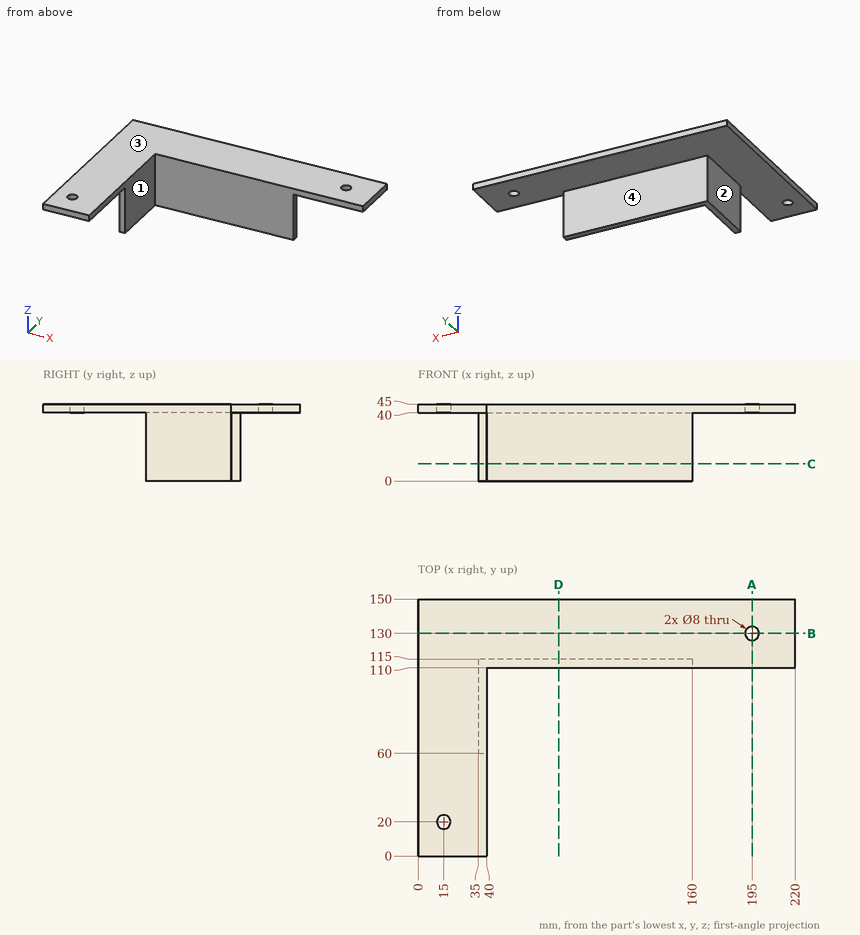
Print and shaded views of the part. All mm, measured from the part's lowest x, y and z. A direction names the side the tool comes from. Give positions to 0.01 mm unless a question says otherwise; leave off trailing zeros. Loops run counter-clockwise (first coordinate to the right, second up) from the corner with the lowest first, then second, coordinate; pieces in that order, holes last. Notation, with made-up numbers: (58.25, 57.25) - (93.25, 57.25) arc R23 cw to (93.25, 82.25) - close; hole circle Ø7 at (-19.75, 58). An arc over 180 degrees is marked (long way). Use a Markdown table: item, result.
(1) Band-saw the part on B-B (y = 130). Give the cut face in (x, z).
Taken from the geometry:
| item | result |
|---|---|
| outline | (0, 40) - (191, 40) - (191, 45) - (0, 45) - close; (199, 40) - (220, 40) - (220, 45) - (199, 45) - close |
(2) Band-saw the part on D-D (x = 82). Give the cut face in (y, z).
Taken from the geometry:
| item | result |
|---|---|
| outline | (110, 0) - (115, 0) - (115, 40) - (150, 40) - (150, 45) - (110, 45) - close |
(3) Band-saw the part on C-C (z = 10). Give the cut face in (x, y).
Taken from the geometry:
| item | result |
|---|---|
| outline | (35, 60) - (40, 60) - (40, 110) - (160, 110) - (160, 115) - (35, 115) - close |
(4) Drop flat-ended pins along their axis: pin 1 Ø10 at (y, z) = (61.5, 27.5) entering from -X; pin 2 Ø2.5 at (x, z) = (37, 24) entering from -Y; pin 3 Ø2 at (x, z) = (58, 6) entering from +Y; pin 4 Ø6.5 at (x, y) = (15, 20) entering from -Z. Give the stop position or say it passes through.
Taken from the geometry:
| item | result |
|---|---|
| pin 1 | x = 35 |
| pin 2 | y = 60 |
| pin 3 | y = 115 |
| pin 4 | through |
(5) Wall check: line 1 along Y through (x, z) = (15, 43); line 2 along Y through (x, z) = (195, 41.9); line 3 along Y through (x, z) = (84, 26). Give the ranges that are in metal, low to high.
Taken from the geometry:
| item | result |
|---|---|
| line 1 | 0 to 16, 24 to 150 |
| line 2 | 110 to 126, 134 to 150 |
| line 3 | 110 to 115 |
(6) Which spindle directions (+Z, -Z, +X, -X, +Y, -Y) get a long thin tool onto all of the face, cutting with end or side? Do the marked faces 1, 2, 3 and 4. Say none if no direction does.
Taken from the geometry:
| item | result |
|---|---|
| face 1 | +Z, -Z, +X, -Y |
| face 2 | -Z, -X, +Y, -Y |
| face 3 | +Z, +X, -X, +Y, -Y |
| face 4 | -Z, +X, -X, +Y |
(7) Band-saw the part on A-A (x = 195). Give the cut face in (y, z).
Taken from the geometry:
| item | result |
|---|---|
| outline | (110, 40) - (126, 40) - (126, 45) - (110, 45) - close; (134, 40) - (150, 40) - (150, 45) - (134, 45) - close |
